Answer from the drawing. Dimensions are ordinates in mm from the lowest x, y and z of the part. A direction names the side the tool comes from. Coordinates: 2 decimals unless noted, no trailing zeros. Order: outer loops, then holes, each group sorted by start corner. A loop starts at its lowest first (then second) coordinate and runs counter-clockwise, first axis right, second up. Notation, with made-up numbers: M 61.5,21.5 L 104.5,21.5 A36 ccw 104.5,55.5 Z; hole C 50,-38 d8. An arc over 180 degrees is marked long. One line per question, with ' | ' between items. Start each with the question number.
1) Find section D-D, the plane y = 52.5. Write down the section's boundary in (x, z).
2) Given P1, Ø10, axis at y = 21.59, z = 68.58, coming from the +X side; P2, Ø1.5, axis at y = 111.5, z = 71.5, coming from the -X side; P3, Ø9, axis at x = 38.1, y = 83.81, coming from the -Z side, each flat-ended and moving along its own axis, determine where each tip first touches the part or whether it passes through.
3) Consider probe 1 along Z at (x, y) = (139.75, 21.59); probe 2 along Y at (x, z) = (38.1, 169.5); probe 3 along X at (y, z) = (7, 156.5). Determine where each line is inside the solid, lowest interval first.
4) A tool of negligible diameter and unlimited length cuts with its end or side. For the marked faces 1 and 2, from which of +Z, -Z, +X, -X, +Y, -Y can it reach the whole face along a straight path? Write none if from no direction.
5) Find section B-B, the plane z = 68.58. Write down the section's boundary in (x, y).
6) Find section C-C, the plane y = 21.59. Write down the section's boundary in (x, z).
7) Find section A-A, the plane x = 38.1. Write down the section's boundary in (y, z).
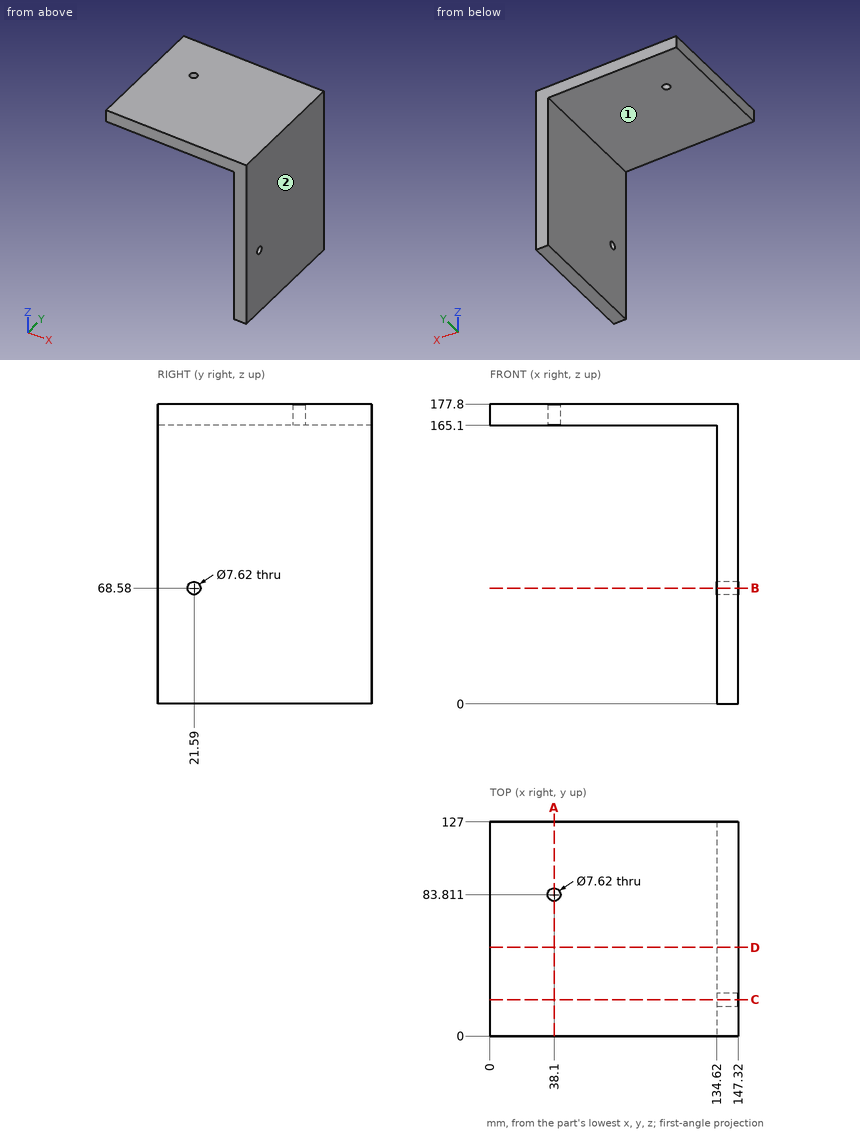
Report:
1) outline: M 0,165.1 L 134.62,165.1 L 134.62,0 L 147.32,0 L 147.32,177.8 L 0,177.8 Z
2) P1: stops at x = 147.32 | P2: stops at x = 134.62 | P3: stops at z = 165.1
3) probe 1: z = 0 to 64.77, 72.39 to 177.8 | probe 2: y = 0 to 80, 87.62 to 127 | probe 3: x = 134.62 to 147.32
4) face 1: -Z, -X, +Y, -Y | face 2: +Z, -Z, +X, +Y, -Y
5) outline: M 134.62,0 L 147.32,0 L 147.32,17.78 L 134.62,17.78 Z; M 134.62,25.4 L 147.32,25.4 L 147.32,127 L 134.62,127 Z
6) outline: M 0,165.1 L 134.62,165.1 L 134.62,72.39 L 147.32,72.39 L 147.32,177.8 L 0,177.8 Z; M 134.62,0 L 147.32,0 L 147.32,64.77 L 134.62,64.77 Z
7) outline: M 0,165.1 L 80,165.1 L 80,177.8 L 0,177.8 Z; M 87.62,165.1 L 127,165.1 L 127,177.8 L 87.62,177.8 Z
